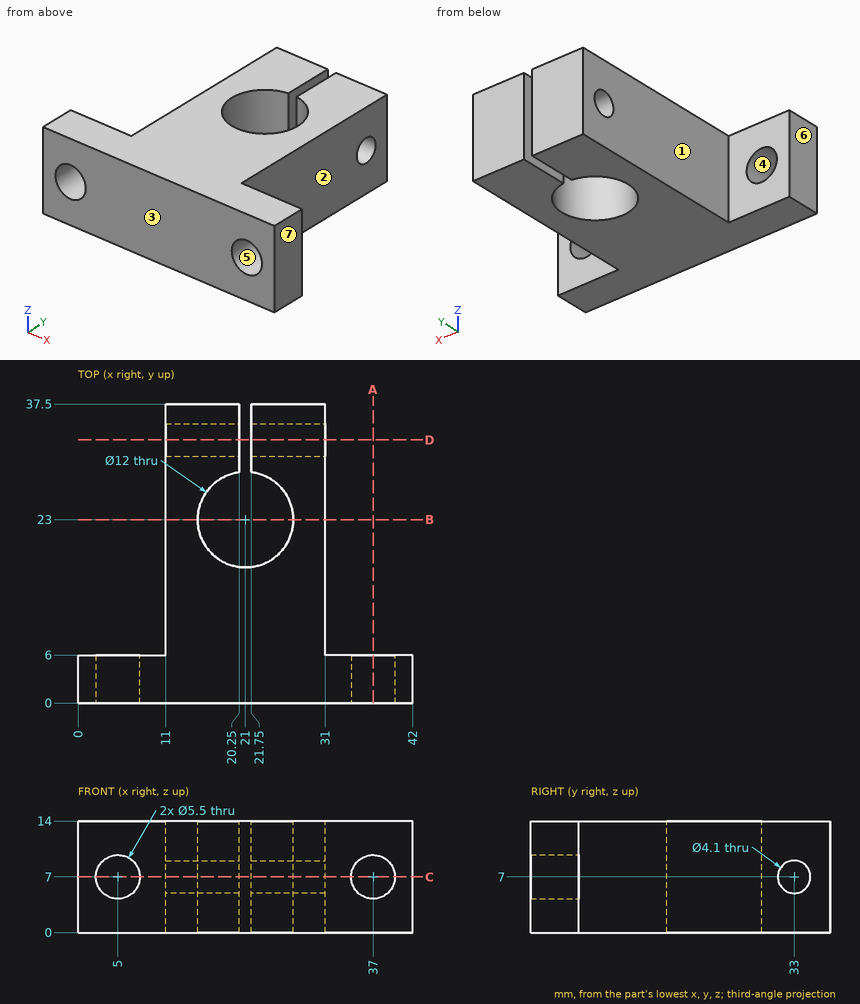
Print and shaded views of the part. All mm, measured from the part's lowest x, y and z. A direction names the side the tool comes from. Give positions to 0.01 mm unless a question says otherwise; leave off trailing zeros. Write each loop counter-clockwise with the first axis right and the second up, starting at its lowest first coordinate (ties: lowest second). Pieces come first, ordered by that corner, then holes. Notation, with made-up numbers: M 44,86 L 100,86 A17 ccw 100,92 Z; hole C 78.5,-9 d10. An arc over 180 degrees is marked long. Use a Markdown table: item, result.
1) Cut at B-B (y = 23). List the corners of the cut face in (x, z), and give its area (3 significant figures).
Responses:
| item | result |
|---|---|
| outline | M 11,0 L 15,0 L 15,14 L 11,14 Z; M 27,0 L 31,0 L 31,14 L 27,14 Z |
| area | 112 mm2 |
2) Cut at D-D (y = 33). List the corners of the cut face in (x, z).
Responses:
| item | result |
|---|---|
| outline | M 11,0 L 20.25,0 L 20.25,4.95 L 11,4.95 Z; M 11,9.05 L 20.25,9.05 L 20.25,14 L 11,14 Z; M 21.75,0 L 31,0 L 31,4.95 L 21.75,4.95 Z; M 21.75,9.05 L 31,9.05 L 31,14 L 21.75,14 Z |
3) Cut at C-C (z = 7). List the corners of the cut face in (x, y).
Responses:
| item | result |
|---|---|
| outline | M 0,0 L 2.25,0 L 2.25,6 L 0,6 Z; M 7.75,0 L 34.25,0 L 34.25,6 L 31,6 L 31,30.95 L 21.75,30.95 L 21.75,28.95 A6 cw long 20.25,28.95 L 20.25,30.95 L 11,30.95 L 11,6 L 7.75,6 Z; M 11,35.05 L 20.25,35.05 L 20.25,37.5 L 11,37.5 Z; M 21.75,35.05 L 31,35.05 L 31,37.5 L 21.75,37.5 Z; M 39.75,0 L 42,0 L 42,6 L 39.75,6 Z |
4) Pull direction X, two halves, no side cores. Call the marked faces 4, 5, 6 and 7: +X half, -X half, draft (parallel to the pull), parting line (faces both ways), or undercut.
Responses:
| item | result |
|---|---|
| face 4 | undercut |
| face 5 | undercut |
| face 6 | -X half |
| face 7 | +X half |
5) Cut at A-A (x = 37). List the corners of the cut face in (y, z).
Responses:
| item | result |
|---|---|
| outline | M 0,0 L 6,0 L 6,4.25 L 0,4.25 Z; M 0,9.75 L 6,9.75 L 6,14 L 0,14 Z |
6) Pin check, flat tips, straight feed: pin 1 (2 mm diameter, centred on y = 29, z = 11.5, fed in from -X); pin 2 (4.5 mm diameter, centred on y = 35, z = 7, fed in from +X); pin 3 (5.5 mm diameter, centred on x = 8, z = 7, fed in from +Y). Stop position of each tip, or through.
Responses:
| item | result |
|---|---|
| pin 1 | stops at x = 11 |
| pin 2 | stops at x = 31 |
| pin 3 | stops at y = 6 |
7) Drill centre lines: line 1 (Y direction, x = 28, z = 7); line 2 (Y direction, x = 26.25, z = 7); line 3 (Z direction, x = 5, y = 3). Where is each one in solid material? Low to high. Write a range as from..to.
Responses:
| item | result |
|---|---|
| line 1 | y = 0..30.95, 35.05..37.5 |
| line 2 | y = 0..20.1, 25.9..30.95, 35.05..37.5 |
| line 3 | z = 0..4.25, 9.75..14 |
8) Tool access for the marked faces 1, 2 and 3: list every direction of +Z, -Z, +X, -X, +Y, -Y with a clear straight run to the whole face (end or side of a thin tool).
Responses:
| item | result |
|---|---|
| face 1 | +Z, -Z, -X, +Y |
| face 2 | +Z, -Z, +X, +Y |
| face 3 | +Z, -Z, +X, -X, -Y |
